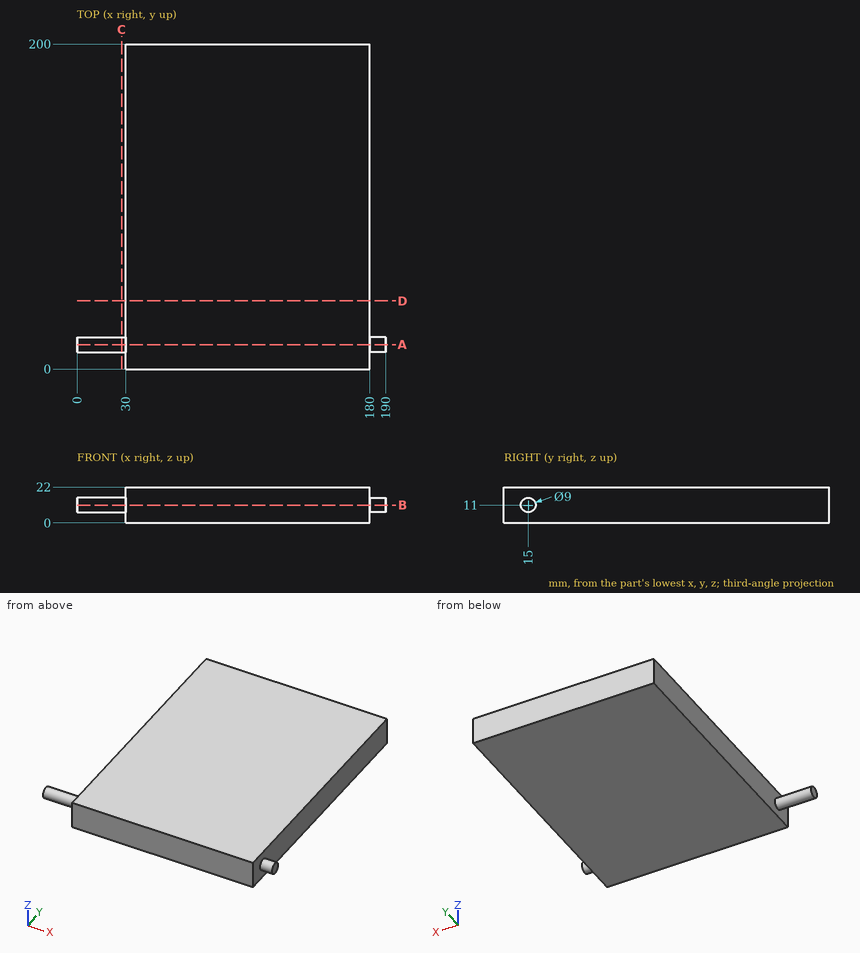
For this review, use the dimensioned drawing (mm, ordinates from the lowest corner) and the shaded views. Give positions to 0.01 mm unless a question says otherwise; leave off trailing zeros. Order: outer loops, then holes, each group sorted by start corner. A loop starts at its lowest first (then second) coordinate and runs counter-clockwise, first axis right, second up.
1. To check wall thickness, follow L1, parallel to X at y = 71, z = 3.5. State the ranges of the line that lie inside material, in increasing order.
Solution:
L1: x = 30 to 180
2. Add section D-D, the plane y = 42. State the section outline as (x, z) points.
Solution:
outline: (30, 0) - (180, 0) - (180, 22) - (30, 22) - close
3. Add section C-C, the plane x = 27.5. State the section outline as (y, z) points, then the cut area to 3 significant figures.
Solution:
outline: circle Ø9 at (15, 11)
area: 63.6 mm2
4. For pin 1 Ø12 at (x, z) = (164.5, 15) entering from -Y; pin 2 Ø2 at (y, z) = (62, 12.5) entering from -X; pin 3 Ø6.5 at (y, z) = (50.5, 15.5) entering from +X, all flat-tipped, find the tip position at first contact; note any pin that passes through.
Solution:
pin 1: stops at y = 0
pin 2: stops at x = 30
pin 3: stops at x = 180
5. Add section A-A, the plane y = 15. State the section outline as (x, z) points.
Solution:
outline: (0, 6.5) - (30, 6.5) - (30, 0) - (180, 0) - (180, 6.5) - (190, 6.5) - (190, 15.5) - (180, 15.5) - (180, 22) - (30, 22) - (30, 15.5) - (0, 15.5) - close
6. Add section B-B, the plane z = 11. State the section outline as (x, y) points, then the cut area to 3 significant figures.
Solution:
outline: (0, 10.5) - (30, 10.5) - (30, 0) - (180, 0) - (180, 10.5) - (190, 10.5) - (190, 19.5) - (180, 19.5) - (180, 200) - (30, 200) - (30, 19.5) - (0, 19.5) - close
area: 30,400 mm2
